Design review of the part shown in the three views and the two pictorial views. Dimensions are in mm from the part's minimum x, y and z. A direction names the side the tool comes from. Coordinates: 2 decimals unless noted, no trailing zeros. Loops run counter-clockwise (first coordinate to the right, second up) from the corner with the lowest first, then second, coordinate; pieces in that order, holes last. Notation, with made-up numbers: (2, 0) -> (9, 0) arc R31 cw to (9, 37) -> close; hole circle Ø3 at (-34, 39). An arc over 180 degrees is marked (long way). One line per item, written item: value.
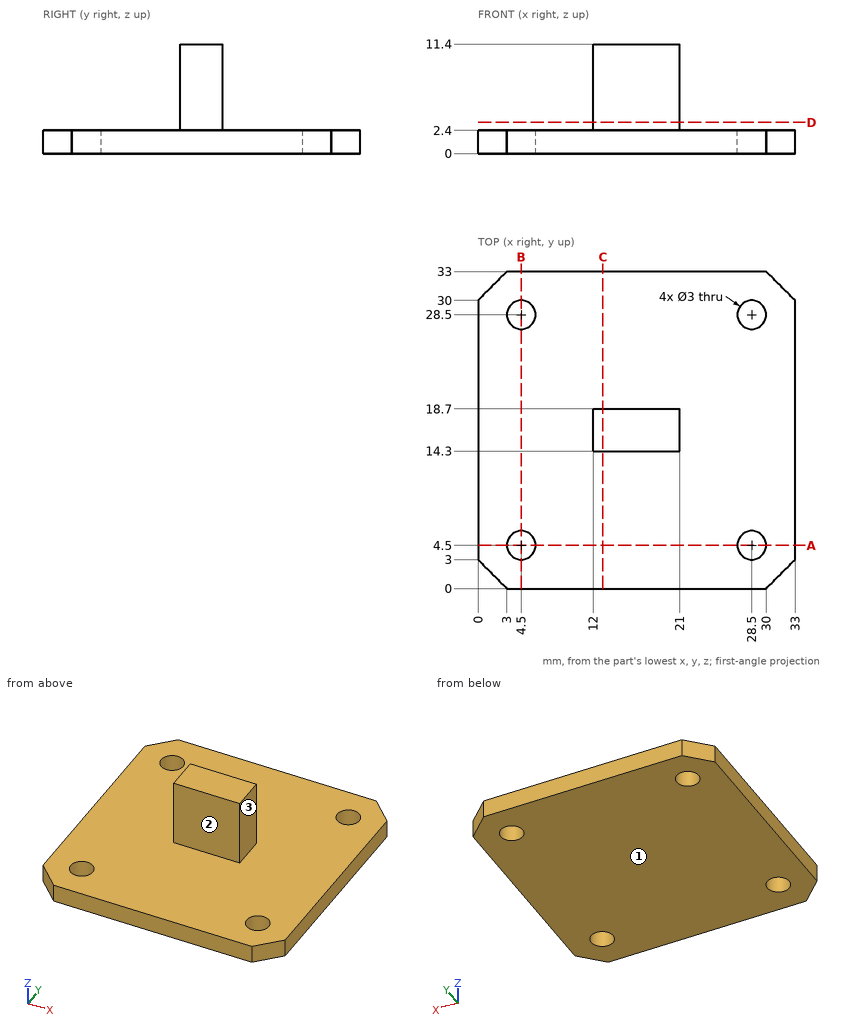
1. To check wall thickness, follow probe 1 along Y at (x, z) = (28.5, 1.6); probe 2 along Z at (x, y) = (3, 15.5); probe 3 along Y at (x, z) = (14.5, 9.75). State the ranges of each line that lie inside material, in increasing order. Write a range as from..to.
Return value:
probe 1: y = 0..3, 6..27, 30..33
probe 2: z = 0..2.4
probe 3: y = 14.3..18.7
2. Take a section at D-D, the plane z = 3.25. Give the boundary of the cut face in (x, y), and give its area (3 significant figures).
Return value:
outline: (12, 14.3) -> (21, 14.3) -> (21, 18.7) -> (12, 18.7) -> close
area: 39.6 mm2
3. Take a section at C-C, the plane x = 13. Give the boundary of the cut face in (y, z).
Return value:
outline: (0, 0) -> (33, 0) -> (33, 2.4) -> (18.7, 2.4) -> (18.7, 11.4) -> (14.3, 11.4) -> (14.3, 2.4) -> (0, 2.4) -> close
4. Take a section at A-A, the plane y = 4.5. Give the boundary of the cut face in (x, z).
Return value:
outline: (0, 0) -> (3, 0) -> (3, 2.4) -> (0, 2.4) -> close; (6, 0) -> (27, 0) -> (27, 2.4) -> (6, 2.4) -> close; (30, 0) -> (33, 0) -> (33, 2.4) -> (30, 2.4) -> close
5. Insertion check: pin 1 Ø1.3 at (y, z) = (15.5, 7.5) entering from -X; pin 2 Ø4.5 at (x, z) = (15.5, 9) entering from +Y; pin 3 Ø5 at (x, y) = (4.5, 28.5) entering from +Z. Each pin has a flat end and moves straight along its axis. Give the tip position at first contact, or say it passes through.
Return value:
pin 1: stops at x = 12
pin 2: stops at y = 18.7
pin 3: stops at z = 2.4
6. For the marked faces 1, 2 and 3, list the 3-axis set-ups (+Z, -Z, +X, -X, +Y, -Y) from which the entire face can be reached by the end or side of a thin tool; tool diameter is ignored.
Return value:
face 1: -Z, +X, -X, +Y, -Y
face 2: +Z, +X, -X, -Y
face 3: +Z, +X, +Y, -Y
